Read the model definition and answer for the solid it produces. Units are mm, in the model's axes. A direction names the side the tool comes from. Coordinates: 2 decimals unless noted, no trailing zeros. Loops run counter-clockwise (first coordinate to the right, second up) from the corner with the lowest first, then second, coordinate; pieces in that order, holes last. Notation, with made-up numbers: (-9, -24.75) -> (-1, -24.75) arc R13 ccw to (-1, -10.75) -> close; hole circle Ø10 at (40, 57). An arc over 180 degrees is marked (long way). Answer in a Markdown table with one row per item.
```python
from build123d import *

# Parameters (mm, degrees)
CROQUIS1_R              = 3.175
SALIENTE_EXTRUIR1_DEPTH = 150
REDONDEO1_R             = 10
CORTAR_EXTRUIR1_DEPTH   = 155.383451186
REDONDEO2_R             = 5
CROQUIS3_W              = 98.791812306
CROQUIS3_H              = 18.145434914
CORTAR_EXTRUIR2_DEPTH   = 155.383451313
CORTAR_EXTRUIR3_DEPTH   = 155.179278889


with BuildPart() as part:
    # Croquis1 → Saliente-Extruir1 (new body)
    with BuildSketch(Plane.XY):
        with BuildLine():
            Line((-3, 19.859827637), (-8.98691391, 23.296314259))
            ThreePointArc((-8.98691391, 23.296314259), (-9.006535925, 33.69237342), (0, 28.5))
            Line((0, 28.5), (0, -28.5))
            ThreePointArc((0, -28.5), (-9.006535925, -33.69237342), (-8.98691391, -23.296314259))
            Line((-8.98691391, -23.296314259), (-3, -19.859827637))
            Line((-3, -19.859827637), (-3, 19.859827637))
        make_face()
        with Locations((-6, 28.5)):
            Circle(CROQUIS1_R, mode=Mode.SUBTRACT)
        with Locations(Location((-6, -28.5, 0), (0, 0, 180))):
            Circle(CROQUIS1_R, mode=Mode.SUBTRACT)
    extrude(amount=-SALIENTE_EXTRUIR1_DEPTH)

    # Redondeo1
    redondeo1_edges = [part.edges().sort_by_distance(p)[0] for p in [
        (-3, -19.859827637, -75),
        (-3, 19.859827637, -75),
    ]]
    fillet(redondeo1_edges, radius=REDONDEO1_R)

    # Croquis2 → Cortar-Extruir1 (cut, through all)
    with BuildSketch(Plane(origin=(0, 0, 0), x_dir=(0, 0, -1), z_dir=(1, 0, 0))):
        Polygon((16, 25), (20, 15.646846929), (20, -15.646846929), (16, -25), (-29.873538988, -25), (-29.873538988, 25), align=None)
    extrude(amount=-CORTAR_EXTRUIR1_DEPTH, mode=Mode.SUBTRACT)

    # Redondeo2
    redondeo2_edges = [part.edges().sort_by_distance(p)[0] for p in [
        (-1.562589533, 15.646846929, -20),
        (-1.562589533, -15.646846929, -20),
        (-5.436698586, -25, -16),
        (-5.436698586, 25, -16),
    ]]
    fillet(redondeo2_edges, radius=REDONDEO2_R)

    # Croquis3 → Cortar-Extruir2 (cut, through all)
    with BuildSketch(Plane(origin=(0, 0, 0), x_dir=(0, 0, -1), z_dir=(1, 0, 0))):
        with Locations((75, 35.875128035)):
            Rectangle(CROQUIS3_W, CROQUIS3_H)
        with Locations((75, -35.875128035)):
            Rectangle(CROQUIS3_W, CROQUIS3_H)
    extrude(amount=-CORTAR_EXTRUIR2_DEPTH, mode=Mode.SUBTRACT)

    # Croquis4 → Cortar-Extruir3 (cut, through all)
    with BuildSketch(Plane.ZY.offset(3)):
        with BuildLine():
            Line((-143.359821197, 2.579074159), (-139.627206237, 2.579074159))
            ThreePointArc((-139.627206237, 2.579074159), (-137.048132079, 0), (-139.627206237, -2.579074159))
            Line((-139.627206237, -2.579074159), (-143.359821197, -2.579074159))
            ThreePointArc((-143.359821197, -2.579074159), (-145.938895356, 0), (-143.359821197, 2.579074159))
        make_face()
    extrude(amount=-CORTAR_EXTRUIR3_DEPTH, mode=Mode.SUBTRACT)


solid = part.part
```
1. A cutting plane is placed at B-B on y = 0.5. Give the vertices of the cut face in (x, z), and give its area (3 significant figures).
A:
| item | result |
|---|---|
| outline | (-3, -150) -> (0, -150) -> (0, -145.89) -> (-3, -145.89) -> close; (-3, -137.1) -> (0, -137.1) -> (0, -20) -> (-3, -20) -> close |
| area | 364 mm2 |
2. The mould has two halves that part along Z. Classify faces 4 (the flat face through (-5, -32, -124.396)), 5 (the cylindrical face through (-5.51, 24.15, -15.49)), 6 (the cylindrical face through (-4.38, 19.14, -84.37)): pulls with the +Z half, pulls with the -Z half, needs draft (parallel to the pull), parting line crosses it, or undercut.
A:
| item | result |
|---|---|
| face 4 | undercut |
| face 5 | pulls with the +Z half |
| face 6 | needs draft |
3. A cutting plane is placed at A-A on z = -135. Give the vertices of the cut face in (x, y) (3 decimals).
A:
| item | result |
|---|---|
| outline | (-8.987, -23.296) arc R6 ccw (long way) to (0, -28.5) -> (0, 28.5) arc R6 ccw (long way) to (-8.987, 23.296) -> (-8.022, 22.742) arc R10 cw to (-3, 14.07) -> (-3, -14.07) arc R10 cw to (-8.022, -22.742) -> close; hole circle Ø6.35 at (-6, -28.5); hole circle Ø6.35 at (-6, 28.5) |
4. Given pin 1 Ø6 at (x, y) = (-5, 31.5) entering from +Z; pin 2 Ø3.5 at (x, y) = (-1, 6.5) entering from +Z; pin 3 Ø3.5 at (x, z) = (-4, -8.5) entering from -Y; pin 4 Ø1.5 at (x, z) = (-2, -141.5) entering from -Y, each flat-ended and moving along its own axis, determine where each tip first touches the part or whether it passes through.
A:
| item | result |
|---|---|
| pin 1 | stops at z = 0 |
| pin 2 | stops at z = -20 |
| pin 3 | stops at y = -34.49 |
| pin 4 | stops at y = -33.54 |
5. Find the intervals of material crossed by probe 1 along Z at (x, y) = (-10.25, -30.5); probe 2 along X at (y, z) = (-14, -65); probe 3 along Y at (x, z) = (-1.75, -141.5), in increasing order.
A:
| item | result |
|---|---|
| probe 1 | z = -150 to -124.4, -25.6 to 0 |
| probe 2 | x = -3 to 0 |
| probe 3 | y = -32.74 to -2.58, 2.58 to 32.74 |
6. A cutting plane is placed at C-C on z = -55. Give the vertices of the cut face in (x, y) (3 decimals).
A:
| item | result |
|---|---|
| outline | (-11.755, -26.802) -> (-8.683, -26.802) arc R3.175 cw to (-3.317, -26.802) -> (0, -26.802) -> (0, 26.802) -> (-3.317, 26.802) arc R3.175 cw to (-8.683, 26.802) -> (-11.755, 26.802) arc R6 ccw to (-8.987, 23.296) -> (-8.022, 22.742) arc R10 cw to (-3, 14.07) -> (-3, -14.07) arc R10 cw to (-8.022, -22.742) -> (-8.987, -23.296) arc R6 ccw to start |
7. A cutting plane is placed at D-D on y = 30. Give the vertices of the cut face in (x, z), and give its area (3 significant figures).
A:
| item | result |
|---|---|
| outline | (-11.81, -150) -> (-8.8, -150) -> (-8.8, -124.4) -> (-11.81, -124.4) -> close; (-11.81, -25.6) -> (-8.8, -25.6) -> (-8.8, 0) -> (-11.81, 0) -> close; (-3.2, -150) -> (-0.19, -150) -> (-0.19, -124.4) -> (-3.2, -124.4) -> close; (-3.2, -25.6) -> (-0.19, -25.6) -> (-0.19, 0) -> (-3.2, 0) -> close |
| area | 308 mm2 |
8. A tool of negligible diameter and unlimited length cuts with its end or side. For faces 1 (the cylindrical face through (-4.3, -19, -84.4)), 2 (the flat face through (-5, -25, -6)), 3 (the flat face through (-2, 26.802, -74)), from which of +Z, -Z, +X, -X, +Y, -Y can it reach the whole face along a straight path? Write none if from no direction.
A:
| item | result |
|---|---|
| face 1 | +Z, -Z, -X |
| face 2 | +Z, +X, -X |
| face 3 | +X, -X, +Y |
